Check sheet for the modelled part. Datum: model origin and axes. Units: mm. A direction names the side the tool comes from. Coordinates: 2 decimals unless noted, no trailing zeros. Loops run counter-clockwise (first coordinate to the right, second up) from the corner with the lowest first, then second, coordinate; pieces in that order, holes last. Notation, with made-up numbers: M 32.25,-10 L 72.25,-10 A15 ccw 72.25,12 Z; hole C -11,79.25 d1. An arc over 180 degrees is marked long. Return JSON: item names as keys, results as strings.
Autodesk Inventor part; units mm, degrees
ref_plane "YZ Plane" through (0, 0, 0) normal (1, 0, 0) x (0, 1, 0)
ref_plane "XZ Plane" through (0, 0, 0) normal (0, 1, 0) x (-1, 0, 0)
ref_plane "XY Plane" through (0, 0, 0) normal (0, 0, 1) x (1, 0, 0)
sketch "Sketch1" plane through (0, 0, 0) normal (0, 0, 1) x (1, 0, 0)
  line L0 (-47.5, 25) -> (47.5, 25)
  line L1 (47.5, 25) -> (47.5, -25)
  line L2 (47.5, -25) -> (-47.5, -25)
  line L3 (-47.5, -25) -> (-47.5, 25)
  line L4 (-47.5, 25) -> (47.5, -25) construction
  line L5 (47.5, 25) -> (-47.5, -25) construction
  point P0 (0, 0)
  dimension "d0" = 50
  dimension "d20" = 95
extrude "Plate1" add sketch "Sketch1" along normal blind 4
sketch "Sketch2" plane through (-43.5, -25, 0) normal (-1, 0, 0) x (0, -1, 0)
  line L0 (-50, 0) -> (0, 0)
  line L1 (0, 0) -> (0, 50)
  line L2 (0, 50) -> (-50, 50)
  line L3 (-50, 50) -> (-50, 0)
edge flange "Flange1" height 50 angle 90 thickness 4 bend radius 4 thickness toward (-1, 0, 0) relief tear relief width 4 relief depth 2 corner gap 4 corner form 0 edges at (-47.5, 0, 4) (47.5, 0, 4) wall of the first edge with corners at (-43.5, 25, 0) (-43.5, -25, 0) (-43.5, -25, 50) (-43.5, 25, 50)
bend "Bend1"
corner "Corner1"
sketch "Sketch3" plane through (0, 0, 0) normal (1, 0, 0) x (0, 1, 0)
  line L0 (25, 8) -> (25, 50)
  line L1 (25, 50) -> (-25, 50)
  line L2 (-25, 50) -> (-25, 8)
  line L3 (-18, 11) -> (18, 11) construction
  line L4 (18, 11) -> (18, 45) construction
  line L5 (18, 45) -> (-18, 45) construction
  line L6 (-18, 45) -> (-18, 11) construction
  line L7 (-18, 11) -> (18, 45) construction
  line L8 (18, 11) -> (-18, 45) construction
  circle A0 centre (18, 45) radius 2.5
  circle A1 centre (-18, 45) radius 2.5
  circle A2 centre (-18, 11) radius 2.5
  circle A3 centre (18, 11) radius 2.5
  point P0 (0, 0)
  point P1 (0, 28)
  dimension "d12" = 5
  dimension "d13" = 7
  dimension "d14" = 7
  dimension "d15" = 34
  dimension "d16" = 5
extrude "Extrusion1" cut sketch "Sketch3" along normal through all both and the other way through all contours A0 | A1
fillet "Fillet1" radius 2 4 edges at (-45.5, 25, 50) (-45.5, -25, 50) (45.5, 25, 50) (45.5, -25, 50)
extrude "Extrusion2" cut sketch "Sketch3" along normal through all contours A2 | A3
equation "\"d14\" = d13"
equation "\"d2\" = BendReliefWidth"
equation "\"d3\" = BendReliefDepth"
equation "\"d4\" = MinimumRemnant"
equation "\"d5\" = BendRadius"
equation "\"d8\" = BendRadius"
equation "\"d9\" = CornerReliefSize"
equation "\"d10\" = GapSize"
equation "\"d11\" = JacobiRadiusSize"
equation "\"BendRadius\" = Thickness"
equation "\"BendReliefWidth\" = Thickness"
equation "\"BendReliefDepth\" = 0.5 * Thickness"
equation "\"CornerReliefSize\" = 4 * Thickness"
equation "\"MinimumRemnant\" = 2 * Thickness"
equation "\"TransitionRadius\" = BendRadius"
equation "\"JacobiRadiusSize\" = BendRadius"
equation "\"GapSize\" = Thickness"
equation "\"d1\" = BendRadius"
properties part number "coluna-apoio" material "Aluminum 6061"
1) Section check B-B on z = 20. Record the cut outline in (x, y), then the cut area to 3 significant figures.
Answers:
{"outline": "M -47.5,-25 L -43.5,-25 L -43.5,25 L -47.5,25 Z; M 43.5,-25 L 47.5,-25 L 47.5,25 L 43.5,25 Z", "area": "400 mm²"}
2) Scan lines: line 1 along Y through (x, z) = (45.65, 11); line 2 along X through (y, z) = (-21.5, 9.5); line 3 along Z through (x, y) = (2, 9.5). Record each from-to range of solid material in increasing order. Write a range as [from, to].
Answers:
{"line 1": "[-25, -20.5], [-15.5, 15.5], [20.5, 25]", "line 2": "[-47.5, -43.5], [43.5, 47.5]", "line 3": "[0, 4]"}
3) Section check C-C on y = 18. Record the cut outline in (x, z).
Answers:
{"outline": "M -47.5,8 A8 ccw -39.5,0 L 39.5,0 A8 ccw 47.5,8 L 47.5,8.5 L 43.5,8.5 L 43.5,8 A4 cw 39.5,4 L -39.5,4 A4 cw -43.5,8 L -43.5,42.5 L -47.5,42.5 Z; M -47.5,47.5 L -43.5,47.5 L -43.5,50 L -47.5,50 Z; M 43.5,13.5 L 47.5,13.5 L 47.5,42.5 L 43.5,42.5 Z; M 43.5,47.5 L 47.5,47.5 L 47.5,50 L 43.5,50 Z"}
4) Section check A-A on z = 11. Record the cut outline in (x, y), then the cut area to 3 significant figures.
Answers:
{"outline": "M -47.5,-25 L -43.5,-25 L -43.5,25 L -47.5,25 Z; M 43.5,-25 L 47.5,-25 L 47.5,-20.5 L 43.5,-20.5 Z; M 43.5,-15.5 L 47.5,-15.5 L 47.5,15.5 L 43.5,15.5 Z; M 43.5,20.5 L 47.5,20.5 L 47.5,25 L 43.5,25 Z", "area": "360 mm²"}
5) Set-up check for faces 5 (the face through (42.359, 0.35, 5.203)), 6 (the face through (45.53, 24.43, 49.4)): record each of +Z, -Z, +X, -X, +Y, -Y from which the full face is reachable in a straight line by a thin tool's end or side.
Answers:
{"face 5": "+Z, +Y, -Y", "face 6": "+Z, +X, -X, +Y"}
6) Go/stop test with flat-tipped pins: pin 1 Ø4 at (y, z) = (-18, 45) entering from -X; pin 2 Ø12 at (x, y) = (11, -5.5) entering from +Z. Record where each tip stops, or that it passes through.
Answers:
{"pin 1": "through", "pin 2": "z = 4"}
7) Draft check along Y on faces 1 (the face through (0, 25, 3)), 2 (the face through (-1, 0, 0)), 3 (the face through (45.5, -20, 46.5)), 4 (the face through (-45.5, -20, 43.5)). Enter one of: +Y half, -Y half, draft (parallel to the pull), parting line (faces both ways), or undercut.
Answers:
{"face 1": "+Y half", "face 2": "draft", "face 3": "undercut", "face 4": "undercut"}
8) Section check D-D on y = -4. Record the cut outline in (x, z).
Answers:
{"outline": "M -47.5,8 A8 ccw -39.5,0 L 39.5,0 A8 ccw 47.5,8 L 47.5,50 L 43.5,50 L 43.5,8 A4 cw 39.5,4 L -39.5,4 A4 cw -43.5,8 L -43.5,50 L -47.5,50 Z"}
